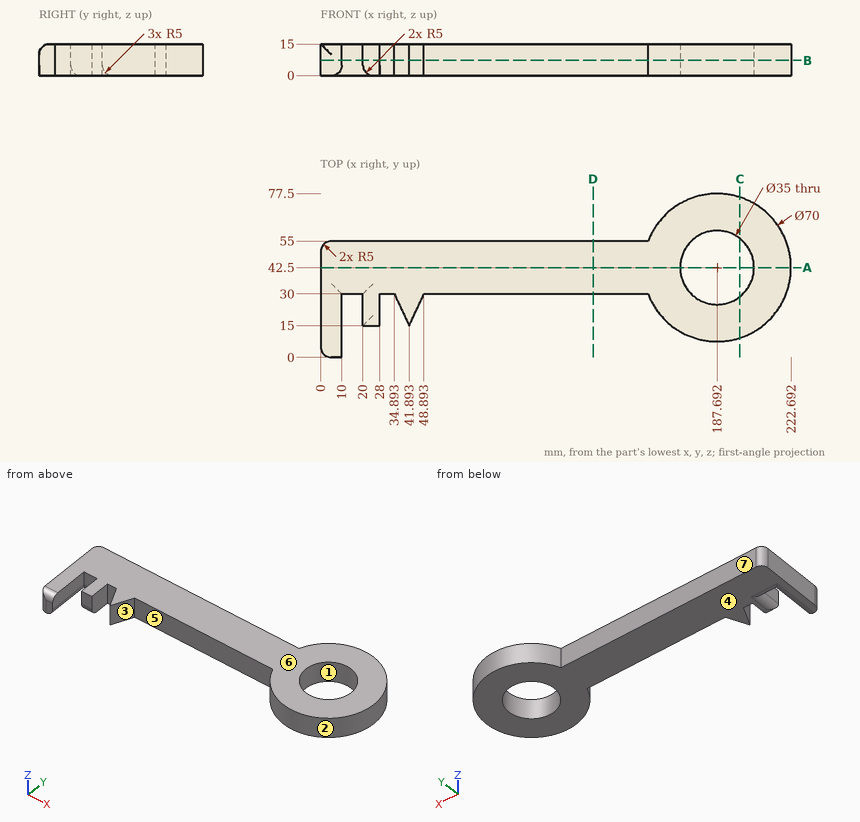
Answer from the drawing. Dimensions are ordinates in mm from the lowest x, y and z of the part. A direction names the side the tool comes from. Round coordinates to 2 decimals unless told otherwise and drop trailing zeros. Loops run counter-clockwise (first coordinate to the right, second up) from the corner with the lowest first, then second, coordinate; pieces in that order, holes last. Notation, with made-up numbers: (48, -24.75) - (68, -24.75) arc R15 cw to (68, -2.75) - close; hole circle Ø10 at (-8.5, 68). An arc over 180 degrees is marked (long way). Return JSON: item names as keys, results as strings. Group by question number.
1. The part is cut by section D-D on x = 129. Determine the outline of the cut face in (y, z).
2. The part is cut by section B-B on z = 7.25. Determine the outline of the cut face in (x, y).
3. Each of these flat-tipped pins is pushed along its axis until it touches: P1, Ø3, axis at y = 51, z = 12.5, coming from the -X side; P2, Ø1, axis at y = 14, z = 7.5, coming from the +X side; P3, Ø1.5, axis at y = 39, z = 3, coming from the +X side; P4, Ø4.5, axis at y = 22, z = 5.5, coming from the +X side. Where does it stop, or does it pass through?
4. The part is cut by section C-C on x = 198.5. Determine the outline of the cut face in (y, z).
5. Which of the six approach directions +Z, -Z, +X, -X, +Y, -Y give full straight-line access (tool end or side, diameter ignored) to the marked faces 5, 6 and 7?
6. Consider probe 1 along X at (y, z) = (23, 6.75) (1 decimal); probe 2 along X at (y, z) = (19, 6.25) (1 decimal); probe 3 along Y at (x, z) = (188, 7). Determine where each line is inside the solid, lowest interval first.
7. The part is cut by section A-A on y = 42.5. Determine the outline of the cut face in (x, z), then the cut area to 3 significant figures.
8. The mould has two halves that part along Y. Classify the marked faces 1, 2, 3 and 4: pulls with the +Y half, pulls with the -Y half, needs draft (parallel to the pull), parting line crosses it, or undercut.
Resolved:
{
 "1": {"outline": "(30, 0) - (55, 0) - (55, 15) - (30, 15) - close"},
 "2": {"outline": "(0, 5) arc R5 ccw to (5, 0) - (10, 0) - (10, 30) - (20, 30) - (20, 15) - (28, 15) - (28, 30) - (34.89, 30) - (41.89, 15) - (48.89, 30) - (155, 30) arc R35 ccw (long way) to (155, 55) - (5, 55) arc R5 ccw to (0, 50) - close; hole circle Ø35 at (187.69, 42.5)"},
 "3": {"P1": "stops at x = 0", "P2": "stops at x = 208.69", "P3": "stops at x = 222.58", "P4": "stops at x = 217.56"},
 "4": {"outline": "(9.21, 0) - (28.74, 0) - (28.74, 15) - (9.21, 15) - close; (56.26, 0) - (75.79, 0) - (75.79, 15) - (56.26, 15) - close"},
 "5": {"face 5": "+Z, -Z, -Y", "face 6": "+Z, +X, -X, +Y, -Y", "face 7": "+Z, -Z, -X, +Y"},
 "6": {"probe 1": "x = 0 to 10, 20 to 28, 38.2 to 45.6, 158.6 to 216.8", "probe 2": "x = 0 to 10, 20 to 28, 40 to 43.8, 161.8 to 213.6", "probe 3": "y = 7.5 to 25, 60 to 77.5"},
 "7": {"outline": "(0, 0) - (170.19, 0) - (170.19, 15) - (0, 15) - close; (205.19, 0) - (222.69, 0) - (222.69, 15) - (205.19, 15) - close", "area": "2,820 mm²"},
 "8": {"face 1": "undercut", "face 2": "parting line crosses it", "face 3": "pulls with the -Y half", "face 4": "needs draft"}
}
